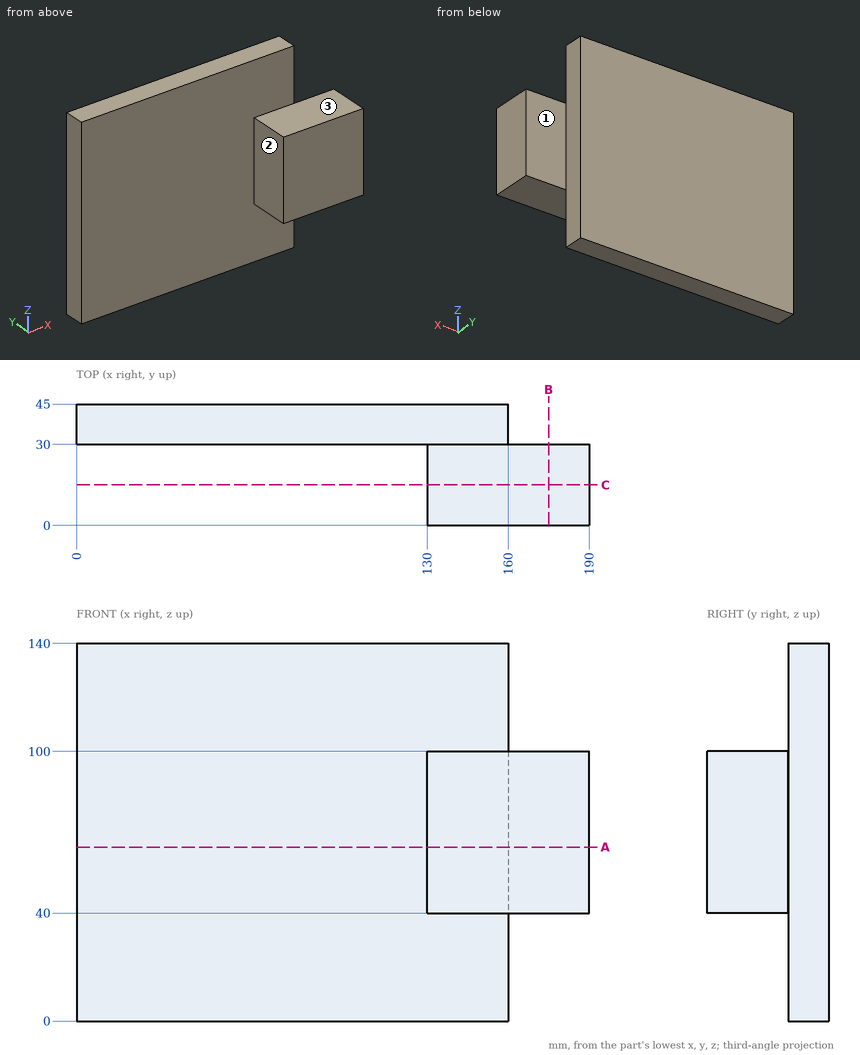
Answer from the drawing. Dimensions are ordinates in mm from the lowest x, y and z of the part. A direction names the side the tool comes from. Give positions to 0.01 mm unless a question says otherwise; leave off trailing zeros. Order: outer loops, then holes, each group sorted by start corner. A loop starts at its lowest first (then second) coordinate and runs counter-clockwise, first axis right, second up. Notation, with made-up numbers: (46.5, 58.5) - (90.5, 58.5) arc R12 ccw to (90.5, 80.5) - close; hole circle Ø10 at (39.5, 56). An arc over 180 degrees is marked (long way). Use one line per item in the form item = value.
1) Each of these flat-tipped pins is pushed along its axis until it touches: pin 1 (6 mm diameter, centred on x = 167.5, y = 11.5, fed in from -Z); pin 2 (12 mm diameter, centred on y = 23.5, z = 116.5, fed in from +X); pin 3 (8 mm diameter, centred on x = 116, z = 51.5, fed in from -Y); pin 4 (7.5 mm diameter, centred on y = 40, z = 48, fed in from +X). Where does it stop, or does it pass through?
Verdict:
pin_1 = 40
pin_2 = through
pin_3 = 30
pin_4 = 160
2) Consider probe 1 along Z at (x, y) = (144, 28.5); probe 2 along X at (y, z) = (23.5, 88.5); probe 3 along Y at (x, z) = (92, 51). Determine where each line is inside the solid, lowest interval first. Write a range as [from, to].
Verdict:
probe_1 = [40, 100]
probe_2 = [130, 190]
probe_3 = [30, 45]
3) For the marked faces 1, 2 and 3, determine the directions among +Z, -Z, +X, -X, +Y, -Y from which every point of the face is accessible in a straight line to the end or side of a thin tool.
Verdict:
face_1 = +Z, -Z, +X, +Y
face_2 = +Z, -Z, -X, -Y
face_3 = +Z, +X, -X, -Y
4) Find section A-A on z = 64.5. Determine the outline of the cut face in (x, y).
Verdict:
outline = (0, 30) - (130, 30) - (130, 0) - (190, 0) - (190, 30) - (160, 30) - (160, 45) - (0, 45) - close
5) Find section C-C on y = 15. Determine the outline of the cut face in (x, z).
Verdict:
outline = (130, 40) - (190, 40) - (190, 100) - (130, 100) - close
6) Find section B-B on x = 175. Determine the outline of the cut face in (y, z), and give its area (3 significant figures).
Verdict:
outline = (0, 40) - (30, 40) - (30, 100) - (0, 100) - close
area = 1,800 mm^2
